```python
from build123d import *

# Parameters (mm, degrees)
CROQUIS1_R              = 1.875
SALIENTE_EXTRUIR1_DEPTH = 6


with BuildPart() as part:
    # Croquis1 → Saliente-Extruir1 (new body)
    with BuildSketch(Plane(origin=(0, 0, 0), x_dir=(1, 0, 0), z_dir=(0, 1, 0))):
        with BuildLine():
            Line((-40, 11), (40, 11))
            ThreePointArc((40, 11), (51, 0), (40, -11))
            Line((40, -11), (-40, -11))
            ThreePointArc((-40, -11), (-51, 0), (-40, 11))
        make_face()
        with Locations((-47, 0)):
            Circle(CROQUIS1_R, mode=Mode.SUBTRACT)
        with Locations((47, 0)):
            Circle(CROQUIS1_R, mode=Mode.SUBTRACT)
        with BuildLine():
            Line((-40, 3), (40, 3))
            ThreePointArc((40, 3), (43, 0), (40, -3))
            Line((40, -3), (-40, -3))
            ThreePointArc((-40, -3), (-43, 0), (-40, 3))
        make_face(mode=Mode.SUBTRACT)
    extrude(amount=SALIENTE_EXTRUIR1_DEPTH)


solid = part.part
```
Can you work these out from the model? Positions are in its coordinate system, mm. A direction names the side the tool comes from. Round coordinates to 2 decimals unless told otherwise and drop trailing zeros. Order: outer loops, then holes, each group sorted by start corner. A loop starts at its lowest first (then second) coordinate and runs counter-clockwise, first axis right, second up. Notation, with made-up numbers: (-15, -25.75) -> (37, -25.75) arc R30 cw to (37, 12.25) -> close; hole circle Ø6 at (32, 1). An arc over 180 degrees is marked (long way). Return JSON: item names as keys, results as strings. Group by question number.
1. Which directions (+Z, -Z, +X, -X, +Y, -Y) give clear straight access to the entire face, cutting with the end or side of a thin tool? Please do faces 1 (the face through (1, 0, -5)), 2 (the face through (-1, 3, -3)).
2. I need wall thicknesses on line 1 (X direction, y = 3.25, z = 0) (3 decimals); line 2 (Z direction, x = 11, y = 2.75); line 3 (X direction, y = 1.95, z = 2). Which ranges of each line are inside material? Lowest first, please. Write a range as [from, to].
3. Will these pins go through, and if not, where does the flat tip stop? pin 1 (1.5 mm diameter, centred on y = 1.5, z = 1.5, fed in from +X); pin 2 (3 mm diameter, centred on y = 4.5, z = 5, fed in from +X).
4. If we section it at A-A, the plane y = 4.05: Write out the boundary of the cut face in (x, z) (3 decimals), then the cut area to 3 significant figures.
5. If we section it at D-D, the plane z = 6.5: Write out the boundary of the cut face in (x, y), then the cut area to 3 significant figures.
6. If we section it at B-B, the plane x = 0: Write out the boundary of the cut face in (y, z), then the cut area to 3 significant figures.
7. If we section it at C-C, the plane x = 47: Write out the boundary of the cut face in (y, z) (3 decimals).
8. We'd pull the mould along X, two halves only. Please class faces 3 (the face through (51, 3, 0)), 4 (the face through (1, 3, 11)), 5 (the face through (43, 3, 0)): released by +X, released by -X, zero draft, split by the parting line, or undercut.
Output values:
{
 "1": {"face 1": "+Z, -Z, +X, -X, -Y", "face 2": "+Y, -Y"},
 "2": {"line 1": "[-51, -48.875], [-45.125, -43], [43, 45.125], [48.875, 51]", "line 2": "[-11, -3], [3, 11]", "line 3": "[-50.82, -42.24], [42.24, 50.82]"},
 "3": {"pin 1": "x = 50.97", "pin 2": "x = 50.43"},
 "4": {"outline": "(-40, -11) -> (40, -11) arc R11 ccw to (40, 11) -> (-40, 11) arc R11 ccw to start; hole circle Ø3.75 at (-47, 0); hole (-40, -3) -> (40, -3) arc R3 ccw to (40, 3) -> (-40, 3) arc R3 ccw to start; hole circle Ø3.75 at (47, 0)", "area": "1,610 mm²"},
 "5": {"outline": "(-48.87, 0) -> (48.87, 0) -> (48.87, 6) -> (-48.87, 6) -> close", "area": "586 mm²"},
 "6": {"outline": "(0, -11) -> (6, -11) -> (6, -3) -> (0, -3) -> close; (0, 3) -> (6, 3) -> (6, 11) -> (0, 11) -> close", "area": "96.0 mm²"},
 "7": {"outline": "(0, -8.485) -> (6, -8.485) -> (6, -1.875) -> (0, -1.875) -> close; (0, 1.875) -> (6, 1.875) -> (6, 8.485) -> (0, 8.485) -> close"},
 "8": {"face 3": "released by +X", "face 4": "zero draft", "face 5": "undercut"}
}
